Could you check a few things on this drawing? It's one solid part, dimensions in mm from its lowest x, y, z. Give positions to 0.01 mm unless a question says otherwise; leave off trailing zeros. Write each loop counter-clockwise with the first axis right and the second up, starting at its lowest first coordinate (ties: lowest second). Pieces come first, ordered by that corner, then holes. Notation, with made-up numbers: M 41,83.25 L 75,83.25 A18 ccw 75,101.25 Z; hole C 59,62.5 d9. An arc over 180 degrees is marked long. Answer as CSV lines item,"result". Start each with the question number.
Q1. Suppose I cut it at A-A (y = 180). Write out the boundary of the cut face in (x, z).
Q2. Suppose I cut it at D-D (z = 0.9). Write out the boundary of the cut face in (x, y).
Q3. If I drill on line 1 along X through (y, z) = (180, 4.05); line 2 along Y through (x, z) = (230, 1.5); line 3 along X through (y, z) = (5, 1.35), over which ranges is the centre line in solid material (lowest first)?
Q4. Suppose I cut it at B-B (y = 5). Write out the boundary of the cut face in (x, z), then the cut area to 3 significant figures.
Q5. For pin 1 (3.5 mm diameter, centred on x = 10, y = 5, fed in from -Z), with a flat end and sliding along its axis, tell me the tip position at first contact or that it passes through.
Q6. Suppose I cut it at C-C (x = 10). Write out the boundary of the cut face in (y, z).
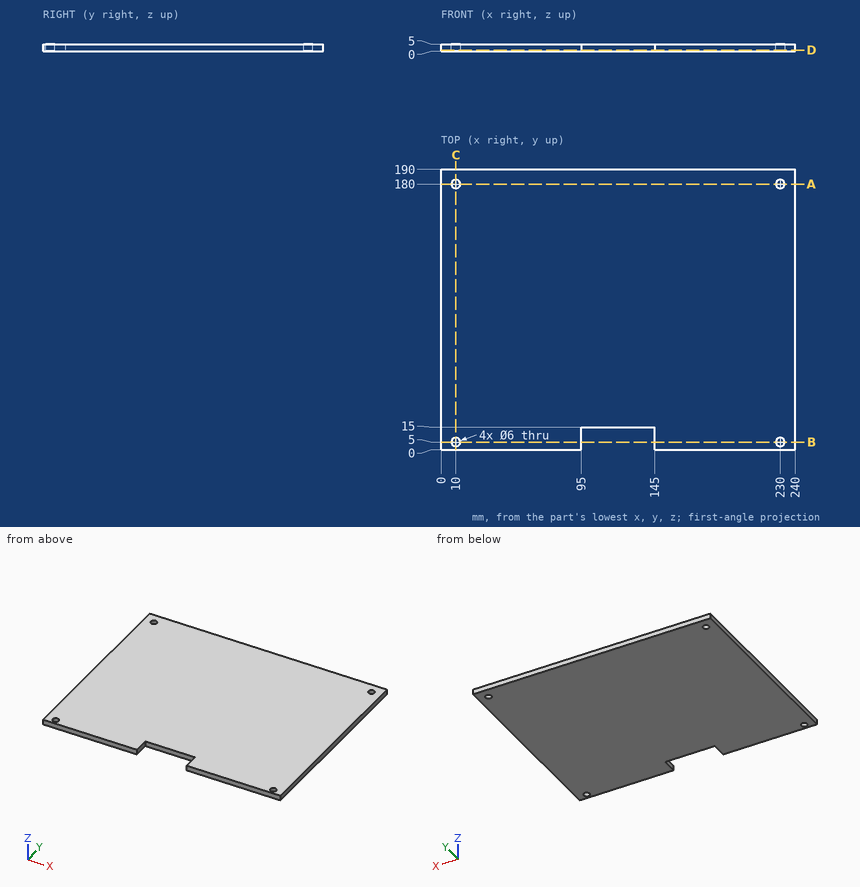
Resolved:
1,outline,"M 0,0 L 7,0 L 7,5 L 0,5 Z; M 13,0 L 227,0 L 227,5 L 13,5 Z; M 233,0 L 240,0 L 240,5 L 233,5 Z"
2,outline,"M 0,0 L 95,0 L 95,15 L 145,15 L 145,0 L 240,0 L 240,190 L 0,190 Z; hole C 10,5 d6; hole C 10,180 d6; hole C 230,5 d6; hole C 230,180 d6"
3,line 1,"0 to 7, 13 to 227, 233 to 240"
3,line 2,"0 to 2, 8 to 177, 183 to 190"
3,line 3,"0 to 7, 13 to 95, 145 to 227, 233 to 240"
4,outline,"M 0,0 L 7,0 L 7,5 L 0,5 Z; M 13,0 L 95,0 L 95,5 L 13,5 Z; M 145,0 L 227,0 L 227,5 L 145,5 Z; M 233,0 L 240,0 L 240,5 L 233,5 Z"
4,area,"890 mm^2"
5,pin 1,"through"
6,outline,"M 0,0 L 2,0 L 2,5 L 0,5 Z; M 8,0 L 177,0 L 177,5 L 8,5 Z; M 183,0 L 190,0 L 190,5 L 183,5 Z"
